Check sheet for the drawn part. Datum: minimum x, y, z corner. Units: mm. A direction names the side the tool comes from. Give positions to 0.01 mm unless a question says otherwise; leave off trailing zeros. Loops run counter-clockwise (first coordinate to the right, second up) from the corner with the lowest first, then second, coordinate; pieces in that order, holes last. Notation, with made-up numbers: (36, 15) - (74, 15) arc R30 ccw to (74, 53) - close; hole circle Ø7 at (62, -20.75). An arc over 180 degrees is marked (long way). Answer in a Markdown table with one row per item.
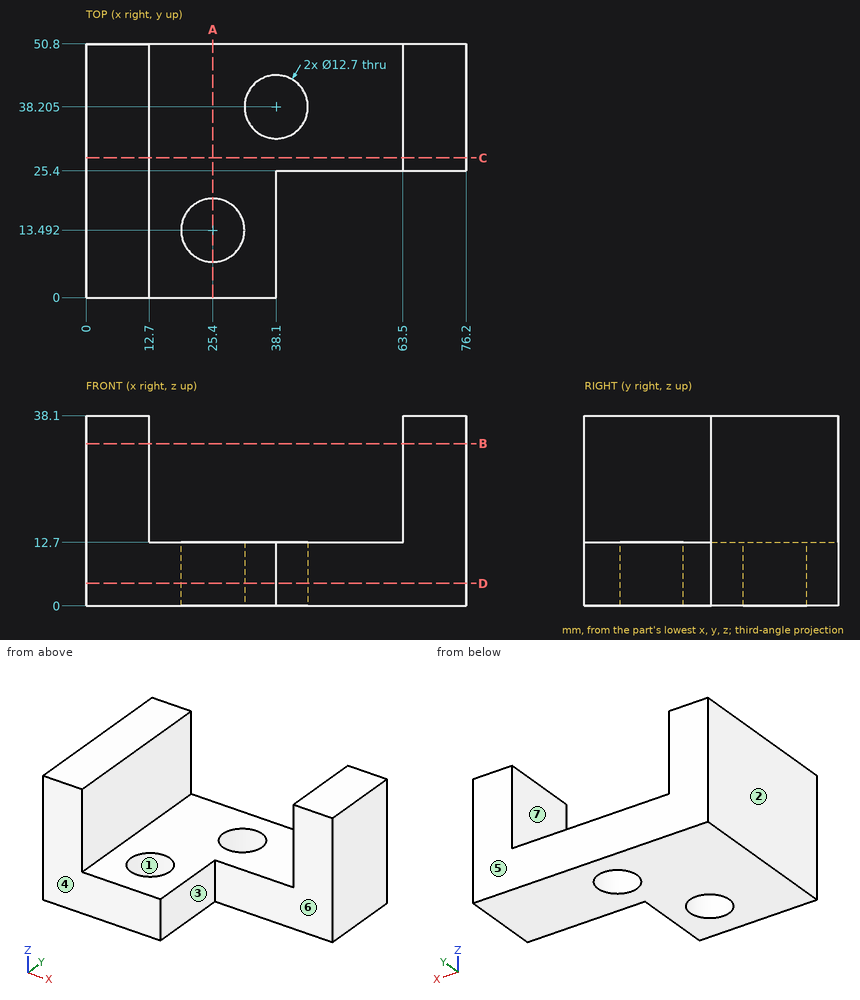
Q1. Tool access check on the marked faces 5, 6 and 7. Record the directions out of +Z, -Z, +X, -X, +Y, -Y that give a thin tool (end or side, any length) a straight path to the whole face; none if there is none.
Completed:
| item | result |
|---|---|
| face 5 | +Z, -Z, +X, -X, +Y |
| face 6 | +Z, -Z, +X, -Y |
| face 7 | +Z, +Y, -Y |
Q2. Sectioned sample at B-B (z = 32.5). Record the cut outline in (x, y).
Completed:
| item | result |
|---|---|
| outline | (0, 0) - (12.7, 0) - (12.7, 50.8) - (0, 50.8) - close; (63.5, 25.4) - (76.2, 25.4) - (76.2, 50.8) - (63.5, 50.8) - close |
Q3. Sectioned sample at C-C (y = 28). Record the cut outline in (x, z), and give its area (3 significant figures).
Completed:
| item | result |
|---|---|
| outline | (0, 0) - (76.2, 0) - (76.2, 38.1) - (63.5, 38.1) - (63.5, 12.7) - (12.7, 12.7) - (12.7, 38.1) - (0, 38.1) - close |
| area | 1,610 mm^2 |
Q4. Sectioned sample at D-D (z = 4.5). Give the number of separate pieces and of enclosed holes in the cut face, and give its area (3 significant figures).
Completed:
| item | result |
|---|---|
| separate pieces | 1 |
| enclosed holes | 2 |
| area | 2,650 mm^2 |
Q5. Draft check along X on the marked faces 1, 2, 3 and 4. Enter one of: +X half, -X half, draft (parallel to the pull), parting line (faces both ways), or undercut.
Completed:
| item | result |
|---|---|
| face 1 | undercut |
| face 2 | -X half |
| face 3 | +X half |
| face 4 | draft |
Q6. Sectioned sample at A-A (x = 25.4). Record the cut outline in (y, z).
Completed:
| item | result |
|---|---|
| outline | (0, 0) - (7.14, 0) - (7.14, 12.7) - (0, 12.7) - close; (19.84, 0) - (50.8, 0) - (50.8, 12.7) - (19.84, 12.7) - close |
Q7. Go/stop test with flat-tipped pins: P1, Ø8, axis at x = 18.5, z = 21.5, coming from the -Y side; P2, Ø15, axis at x = 46.5, y = 26.5, coming from the +Z side; P3, Ø14.5, axis at x = 38.1, y = 38.2, coming from the -Z side; P4, Ø7.5, axis at y = 17.5, z = 27, coming from the +X side. Record where each tip stops, or that it passes through.
Completed:
| item | result |
|---|---|
| P1 | through |
| P2 | z = 12.7 |
| P3 | z = 0 |
| P4 | x = 12.7 |
Q8. Thickness scan on line 1 (X direction, y = 33, z = 33.5); line 2 (Y direction, x = 25.4, z = 4.5); line 3 (Y direction, x = 25, z = 8) (1 decimal). Record the ranges inside material, lowest first.
Completed:
| item | result |
|---|---|
| line 1 | 0 to 12.7, 63.5 to 76.2 |
| line 2 | 0 to 7.14, 19.84 to 50.8 |
| line 3 | 0 to 7.2, 19.8 to 50.8 |
